from build123d import *

# Parameters (mm, degrees)
SKETCH1_R           = 150
BOSS_EXTRUDE1_DEPTH = 10
SKETCH2_R           = 2
CUT_EXTRUDE1_DEPTH  = 10


with BuildPart() as part:
    # Sketch1 → Boss-Extrude1 (new body)
    with BuildSketch(Plane(origin=(0, 0, 0), x_dir=(1, 0, 0), z_dir=(0, 1, 0))):
        Circle(SKETCH1_R)
    extrude(amount=BOSS_EXTRUDE1_DEPTH)

    # Sketch2 → Cut-Extrude1 (cut)
    with BuildSketch(Plane(origin=(0, 10, 0), x_dir=(1, 0, 0), z_dir=(0, 1, 0))):
        with Locations((-14.945, 131.706442493)):
            Circle(SKETCH2_R)
        with Locations((-14.945, 107.646442493)):
            Circle(SKETCH2_R)
        with Locations((14.945, 107.646442493)):
            Circle(SKETCH2_R)
        with Locations((14.945, 131.706442493)):
            Circle(SKETCH2_R)
        with Locations((85.752053826, -66.765970906)):
            Circle(SKETCH2_R)
        with Locations((100.697053826, -40.880471587)):
            Circle(SKETCH2_R)
        with Locations((106.588625041, -78.795970906)):
            Circle(SKETCH2_R)
        with Locations((121.533625041, -52.910471587)):
            Circle(SKETCH2_R)
        with Locations((-100.697053826, -40.880471587)):
            Circle(SKETCH2_R)
        with Locations((-85.752053826, -66.765970906)):
            Circle(SKETCH2_R)
        with Locations((-121.533625041, -52.910471587)):
            Circle(SKETCH2_R)
        with Locations((-106.588625041, -78.795970906)):
            Circle(SKETCH2_R)
    extrude(amount=-CUT_EXTRUDE1_DEPTH, mode=Mode.SUBTRACT)


solid = part.part
Read the model definition and answer for the solid it produces. Units are mm, in the model's axes. Coordinates: 2 decimals unless noted, no trailing zeros. Loops run counter-clockwise (first coordinate to the right, second up) from the corner with the lowest first, then second, coordinate; pieces in that order, holes last.
Q1. Each of these flat-tipped pins is pushed along its axis until it touches: pin 1 Ø5 at (x, y) = (116.5, 7.5) entering from +Z; pin 2 Ø5 at (x, y) = (-106, 5) entering from +Z. Where does it stop, or does it pass through?
Q2. The part is cut by section A-A on y = 5.5. Give the number of separate pieces and of enclosed holes in the cut face, and give its area (3 significant figures).
Q3. The part is cut by section B-B on z = -122. Write down the section's boundary in (x, y).
Q4. Consider probe 1 along X at (y, z) = (1, 42.5); probe 2 along Z at (x, y) = (-16.5, 3.25); probe 3 along Z at (x, y) = (16, 8.25). Determine where each line is inside the solid, lowest interval first.
Q5. The part is cut by section C-C on x = 32. Write down the section's boundary in (y, z).
Results below:
1. pin 1: stops at z = 97.49
1. pin 2: stops at z = 108.57
2. separate pieces: 1
2. enclosed holes: 12
2. area: 70,500 mm2
3. outline: (-87.27, 0) - (87.27, 0) - (87.27, 10) - (-87.27, 10) - close
4. probe 1: x = -143.85 to -101.87, -99.52 to 99.52, 101.87 to 143.85
4. probe 2: z = -149.09 to -132.96, -130.45 to -108.9, -106.39 to 149.09
4. probe 3: z = -149.14 to -133.41, -130.01 to -109.35, -105.95 to 149.14
5. outline: (0, -146.55) - (10, -146.55) - (10, 146.55) - (0, 146.55) - close
